The figure shows three views and two pictorial views of one solid part (mm, origin at its lowest corner). Answer the questions. A direction names the side the tool comes from. Coordinates: 2 decimals unless noted, no trailing zeros. Order: outer loops, then holes, each group sorted by start corner. A loop starts at its lowest first (then second) coordinate and runs counter-clockwise, first axis right, second up. Notation, with made-up numbers: (76.25, 37.25) -> (132.25, 37.25) arc R23 cw to (132.25, 50.25) -> close; hole circle Ø6 at (4.5, -16.75). An arc over 180 degrees is marked (long way). Write item = value, one per line. Start each with the question number.
Q1. The part is cut by section B-B, the plane y = 45. Determine the outline of the cut face in (x, z).
Q2. The part is cut by section A-A, the plane z = 7.5. Determine the outline of the cut face in (x, y), plus the area to 3 significant figures.
Q3. Straight lines are drawn through the part: L1, parallel to X at y = 3.5, z = 7.75; L2, parallel to Z at x = 7.5, y = 5.5; L3, parallel to Y at x = 43.5, z = 7.5. For each, find the intervals that lie inside material, in ascending order. Write a range as from..to.
Q4. The part is cut by section D-D, the plane z = 12.5. Determine the outline of the cut face in (x, y), plus the area to 3 significant figures.
Q5. The part is cut by section C-C, the plane x = 7.5. Determine the outline of the cut face in (y, z), plus the area to 3 significant figures.
Q6. Which of the six approach directions +Z, -Z, +X, -X, +Y, -Y give full straight-line access (tool end or side, diameter ignored) to the marked faces 1 and 2?
Q7. Flat-ended cylindrical pins translate along their axes: pin 1 (2 mm diameter, centred on x = 21, z = 3, fed in from -Y); pin 2 (5 mm diameter, centred on x = 79.5, z = 7.5, fed in from +Y); pin 3 (4.5 mm diameter, centred on y = 47, z = 11, fed in from +X). Find the tip coordinate at first contact, or state that the pin passes through.
Q8. For a pull along X with two mould halves and no side action, classify the marked faces 3, 4, 5 and 6 as +X half, -X half, draft (parallel to the pull), parting line (faces both ways), or undercut.
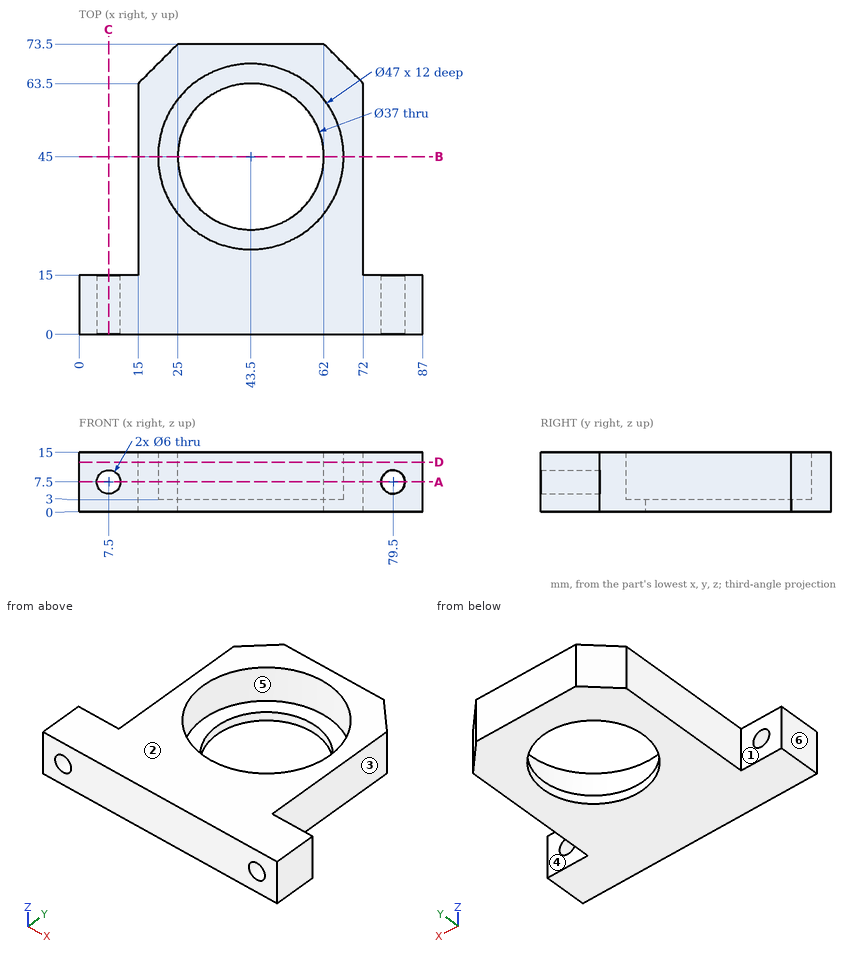
Model answer:
q1.outline = (15, 0) -> (25, 0) -> (25, 3) -> (20, 3) -> (20, 15) -> (15, 15) -> close; (62, 0) -> (72, 0) -> (72, 15) -> (67, 15) -> (67, 3) -> (62, 3) -> close
q2.outline = (0, 0) -> (4.5, 0) -> (4.5, 15) -> (0, 15) -> close; (10.5, 0) -> (76.5, 0) -> (76.5, 15) -> (72, 15) -> (72, 63.5) -> (62, 73.5) -> (25, 73.5) -> (15, 63.5) -> (15, 15) -> (10.5, 15) -> close; (82.5, 0) -> (87, 0) -> (87, 15) -> (82.5, 15) -> close; hole circle Ø47 at (43.5, 45)
q2.area = 2,620 mm2
q3.L1 = 0..4.51, 10.49..76.51, 82.49..87
q3.L2 = 0..4.5, 10.5..15
q3.L3 = 0..21.5, 68.5..73.5
q4.outline = (0, 0) -> (87, 0) -> (87, 15) -> (72, 15) -> (72, 63.5) -> (62, 73.5) -> (25, 73.5) -> (15, 63.5) -> (15, 15) -> (0, 15) -> close; hole circle Ø47 at (43.5, 45)
q4.area = 2,800 mm2
q5.outline = (0, 0) -> (15, 0) -> (15, 4.5) -> (0, 4.5) -> close; (0, 10.5) -> (15, 10.5) -> (15, 15) -> (0, 15) -> close
q5.area = 135 mm2
q6.face_1 = +Z, -Z, -X, +Y
q6.face_2 = +Z, +X, -X, +Y, -Y
q7.pin_1 = 0
q7.pin_2 = through
q7.pin_3 = 72
q8.face_3 = +X half
q8.face_4 = draft
q8.face_5 = undercut
q8.face_6 = -X half
